```python
from build123d import *

# Parameters (mm, degrees)
PAD_DEPTH = 5


with BuildPart() as part:
    # Sketch → Pad (new body)
    with BuildSketch(Plane.XY):
        with BuildLine():
            Line((121.25, 46.5), (121.25, 76.5))
            Line((121.25, 76.5), (91.25, 76.5))
            Line((91.25, 76.5), (91.25, 71.5))
            Line((91.25, 71.5), (-91.25, 71.5))
            Line((-91.25, 71.5), (-91.25, 76.5))
            Line((-91.25, 76.5), (-121.25, 76.5))
            Line((-121.25, 76.5), (-121.25, 32))
            Line((-121.25, 32), (-100.75, 32))
            ThreePointArc((-100.75, -6), (-81.75, 13), (-100.75, 32))
            Line((-100.75, -6), (-121.25, -6))
            Line((-121.25, -6), (-121.25, -76.5))
            Line((-121.25, -76.5), (-91.25, -76.5))
            Line((-91.25, -76.5), (-91.25, -71.5))
            Line((-91.25, -71.5), (91.25, -71.5))
            Line((91.25, -71.5), (91.25, -76.5))
            Line((91.25, -76.5), (121.25, -76.5))
            Line((121.25, -76.5), (121.25, -46.5))
            Line((121.25, -46.5), (126.25, -46.5))
            Line((126.25, -46.5), (126.25, 46.5))
            Line((126.25, 46.5), (121.25, 46.5))
        make_face()
    extrude(amount=PAD_DEPTH)


solid = part.part
```
The model under review builds one solid part; all positions refer to its coordinate system, in mm. A direction names the side the tool comes from. Give positions to 0.01 mm unless a question says otherwise; leave off trailing zeros. Write each loop counter-clockwise with the first axis right and the second up, starting at its lowest first coordinate (ties: lowest second). Pieces come first, ordered by that corner, then holes. Notation, with made-up numbers: (76, 31) -> (123, 31) arc R6 ccw to (123, 35) -> close; hole circle Ø2 at (61, 62.25). An arc over 180 degrees is marked (long way). Put each result on its own line as item: value.
(1) To check wall thickness, follow probe 1 along Y at (x, z) = (-101, 3.3); probe 2 along X at (y, z) = (13, 0.95); probe 3 along Y at (x, z) = (-34, 3.15). State the ranges of each line that lie inside material, in increasing order. Write a range as from..to.
Results are:
probe 1: -76.5..-6, 32..76.5
probe 2: -81.75..126.25
probe 3: -71.5..71.5
(2) For pin 1 Ø2.5 at (y, z) = (-73.5, 3) entering from +X; pin 2 Ø2.5 at (x, z) = (123.5, 2.5) entering from -Y; pin 3 Ø2.5 at (x, z) = (-9, 1.5) entering from -Y, all flat-tipped, find the tip position at first contact; note any pin that passes through.
Results are:
pin 1: x = 121.25
pin 2: y = -46.5
pin 3: y = -71.5
(3) We need section C-C, the plane x = 8.5. Give the boundary of the cut face in (y, z), and give its area (3 significant figures).
Results are:
outline: (-71.5, 0) -> (71.5, 0) -> (71.5, 5) -> (-71.5, 5) -> close
area: 715 mm²
(4) We need section A-A, the plane z = 1.45. Give the boundary of the cut face in (x, y).
Results are:
outline: (-121.25, -76.5) -> (-91.25, -76.5) -> (-91.25, -71.5) -> (91.25, -71.5) -> (91.25, -76.5) -> (121.25, -76.5) -> (121.25, -46.5) -> (126.25, -46.5) -> (126.25, 46.5) -> (121.25, 46.5) -> (121.25, 76.5) -> (91.25, 76.5) -> (91.25, 71.5) -> (-91.25, 71.5) -> (-91.25, 76.5) -> (-121.25, 76.5) -> (-121.25, 32) -> (-100.75, 32) arc R19 cw to (-100.75, -6) -> (-121.25, -6) -> close
(5) Tool access review of faces 5 (the flat face through (-111, 32, 2)), 6 (the flat face through (91.25, -74, 2)), 7 (the flat face through (124, -46.5, 2)), 8 (the flat face through (121.25, 61, 2)), 9 (the flat face through (91.25, 74, 2)): name each direction out of +Z, -Z, +X, -X, +Y, -Y from which nothing blocks a thin tool from reaching the whole face with its end or side.
Results are:
face 5: +Z, -Z, -X
face 6: +Z, -Z, -Y
face 7: +Z, -Z, +X, -Y
face 8: +Z, -Z, +X, +Y
face 9: +Z, -Z, +Y
(6) The part is to be moulded in two halves that separate along Y. For faces 1 (the flat face through (-1, -71.5, 2)), 2 (the flat face through (-106, 76.5, 2)), 3 (the flat face through (-91.25, 74, 2)), 4 (the flat face through (-111, -6, 2)), say which applies: pulls with the +Y half, pulls with the -Y half, needs draft (parallel to the pull), parting line crosses it, or undercut.
Results are:
face 1: pulls with the -Y half
face 2: pulls with the +Y half
face 3: needs draft
face 4: undercut
(7) We need section B-B, the plane y = 13. Give the boundary of the cut face in (x, z).
Results are:
outline: (-81.75, 0) -> (126.25, 0) -> (126.25, 5) -> (-81.75, 5) -> close
